from build123d import *

# Parameters (mm, degrees)
SKETCH1_W               = 95.2
SKETCH1_H               = 135.7
BOSS_EXTRUDE1_DEPTH     = 240
SKETCH3_W               = 228.6
SKETCH3_H               = 83.8
CUT_EXTRUDE1_DEPTH      = 124.3
FILLET1_R               = 1
SKETCH6_R               = 23.5
CUT_EXTRUDE2_DEPTH      = 140
SKETCH7_W               = 55
SKETCH7_H               = 45.7
BOSS_EXTRUDE2_DEPTH     = 8.3
SKETCH8_R               = 23.5
CUT_EXTRUDE3_DEPTH      = 295.494040687
SKETCH9_W               = 55
SKETCH9_H               = 45.7
BOSS_EXTRUDE3_DEPTH     = 8.3
SKETCH10_R              = 23.5
CUT_EXTRUDE4_DEPTH      = 298.512571163
CUT_EXTRUDE5_DEPTH      = 295.494040687
CUT_EXTRUDE5_DEPTH_BACK = 295.494040687
SKETCH11_R              = 4
SKETCH12_W              = 46
SKETCH12_H              = 10
BOSS_EXTRUDE4_DEPTH     = 2
SKETCH13_W              = 46
SKETCH13_H              = 10
BOSS_EXTRUDE5_DEPTH     = 2


with BuildPart() as part:
    # Sketch1 → Boss-Extrude1 (new body)
    with BuildSketch(Plane(origin=(0, 0, 0), x_dir=(0, 0, -1), z_dir=(1, 0, 0))):
        with Locations((47.6, 67.85)):
            Rectangle(SKETCH1_W, SKETCH1_H)
    extrude(amount=-BOSS_EXTRUDE1_DEPTH)

    # Sketch3 → Cut-Extrude1 (cut)
    with BuildSketch(Plane(origin=(0, 135.7, 0), x_dir=(1, 0, 0), z_dir=(0, 1, 0))):
        with Locations((-120, 47.6)):
            Rectangle(SKETCH3_W, SKETCH3_H)
    extrude(amount=-CUT_EXTRUDE1_DEPTH, mode=Mode.SUBTRACT)

    # Fillet1
    fillet1_edges = [part.edges().sort_by_distance(p)[0] for p in [
        (-240, 67.85, -95.2),
        (-240, 67.85, 0),
        (0, 67.85, -95.2),
        (0, 0, -47.6),
        (0, 67.85, 0),
        (-120, 0, -95.2),
        (-120, 0, 0),
        (-240, 0, -47.6),
    ]]
    fillet(fillet1_edges, radius=FILLET1_R)

    # Sketch6 → Cut-Extrude2 (cut)
    with BuildSketch(Plane.XY):
        with Locations((-120, 117.5)):
            Circle(SKETCH6_R)
    extrude(amount=-CUT_EXTRUDE2_DEPTH, mode=Mode.SUBTRACT)

    # Sketch7 → Boss-Extrude2 (add)
    with BuildSketch(Plane.XY):
        with Locations((-120, 112.85)):
            Rectangle(SKETCH7_W, SKETCH7_H)
    extrude(amount=BOSS_EXTRUDE2_DEPTH)

    # Sketch8 → Cut-Extrude3 (cut, through all)
    with BuildSketch(Plane(origin=(0, 0, -95.2), x_dir=(-1, 0, 0), z_dir=(0, 0, -1))):
        with Locations((120, 117.5)):
            Circle(SKETCH8_R)
    extrude(amount=-CUT_EXTRUDE3_DEPTH, mode=Mode.SUBTRACT)

    # Sketch9 → Boss-Extrude3 (add)
    with BuildSketch(Plane(origin=(0, 0, -95.2), x_dir=(-1, 0, 0), z_dir=(0, 0, -1))):
        with Locations((120, 112.85)):
            Rectangle(SKETCH9_W, SKETCH9_H)
    extrude(amount=BOSS_EXTRUDE3_DEPTH)

    # Sketch10 → Cut-Extrude4 (cut, through all)
    with BuildSketch(Plane.XY.offset(8.3)):
        with Locations((-120, 117.5)):
            Circle(SKETCH10_R)
    extrude(amount=-CUT_EXTRUDE4_DEPTH, mode=Mode.SUBTRACT)

    # Sketch11 → Cut-Extrude5 (cut, two sides: drawn at the far end of the back side and taken through both)
    with BuildSketch(Plane.XY.offset(-CUT_EXTRUDE5_DEPTH_BACK)):
        with Locations((-30, 128.7)):
            Circle(SKETCH11_R)
        with Locations((-210, 128.7)):
            Circle(SKETCH11_R)
    extrude(amount=CUT_EXTRUDE5_DEPTH + CUT_EXTRUDE5_DEPTH_BACK, mode=Mode.SUBTRACT)

    # Sketch12 → Boss-Extrude4 (add)
    with BuildSketch(Plane.XY.offset(8.3)):
        with Locations((-120, 97)):
            Rectangle(SKETCH12_W, SKETCH12_H)
    extrude(amount=BOSS_EXTRUDE4_DEPTH)

    # Sketch13 → Boss-Extrude5 (add)
    with BuildSketch(Plane(origin=(0, 0, -103.5), x_dir=(-1, 0, 0), z_dir=(0, 0, -1))):
        with Locations((120, 97)):
            Rectangle(SKETCH13_W, SKETCH13_H)
    extrude(amount=BOSS_EXTRUDE5_DEPTH)


solid = part.part
Geometry check sheet. Reference: the model listing, model coordinates, mm. A direction names the side the tool comes from. Coordinates: 2 decimals unless noted, no trailing zeros. Order: outer loops, then holes, each group sorted by start corner. A loop starts at its lowest first (then second) coordinate and runs counter-clockwise, first axis right, second up. Notation, with made-up numbers: M -12.5,38 L 28.5,38 A18 ccw 28.5,43 Z; hole C 68,-31.5 d9. An arc over 180 degrees is marked long. Use CSV: the item, a comma, the result in double quotes.
Item 1: Gauge pin test, flat ends, axial feed: pin 1 Ø9 at (y, z) = (123.5, -101) entering from +X; pin 2 Ø1 at (x, z) = (-111.5, -104) entering from +Y; pin 3 Ø6 at (x, y) = (-208.5, 94) entering from -Z. Record the tip position at first contact, or that the pin passes through.
Returned:
pin 1,"stops at x = -92.5"
pin 2,"stops at y = 102"
pin 3,"stops at z = -95.2"
Item 2: Cross-section at D-D on x = -217. Record the cut outline in (y, z).
Returned:
outline,"M 0,-94.2 A1 ccw 1,-95.2 L 135.7,-95.2 L 135.7,-89.5 L 11.4,-89.5 L 11.4,-5.7 L 135.7,-5.7 L 135.7,0 L 1,0 A1 ccw 0,-1 Z"
Item 3: Cross-section at A-A on y = 117.5. Record the cut outline in (x, z).
Returned:
outline,"M -240,-94.2 A1 ccw -239,-95.2 L -147.5,-95.2 L -147.5,-103.5 L -143.5,-103.5 L -143.5,-89.5 L -234.3,-89.5 L -234.3,-5.7 L -143.5,-5.7 L -143.5,8.3 L -147.5,8.3 L -147.5,0 L -239,0 A1 ccw -240,-1 Z; M -96.5,-103.5 L -92.5,-103.5 L -92.5,-95.2 L -1,-95.2 A1 ccw 0,-94.2 L 0,-1 A1 ccw -1,0 L -92.5,0 L -92.5,8.3 L -96.5,8.3 L -96.5,-5.7 L -5.7,-5.7 L -5.7,-89.5 L -96.5,-89.5 Z"
Item 4: Cross-section at B-B on x = -30. Record the cut outline in (y, z), then the cut area to 3 significant figures.
Returned:
outline,"M 0,-94.2 A1 ccw 1,-95.2 L 124.7,-95.2 L 124.7,-89.5 L 11.4,-89.5 L 11.4,-5.7 L 124.7,-5.7 L 124.7,0 L 1,0 A1 ccw 0,-1 Z; M 132.7,-95.2 L 135.7,-95.2 L 135.7,-89.5 L 132.7,-89.5 Z; M 132.7,-5.7 L 135.7,-5.7 L 135.7,0 L 132.7,0 Z"
area,"2,410 mm2"
Item 5: Tool access check on faces 4 (the flat face through (-5.7, 74, -47)), 5 (the flat face through (-147.5, 113, 4)), 6 (the cylindrical face through (-120.808, 94.014, -96.402)). Record the directions out of +Z, -Z, +X, -X, +Y, -Y that give a thin tool (end or side, any length) a straight path to the whole face; none if there is none.
Returned:
face 4,"+Y"
face 5,"+Z, -X, +Y, -Y"
face 6,"none"
Item 6: Thickness scan on line 1 along Z through (x, y) = (-38, 53.5); line 2 along X through (y, z) = (65, -27.5); line 3 along Y through (x, z) = (-30, -4.3). Record the ranges inside material, lowest first.
Returned:
line 1,"z = -95.2 to -89.5, -5.7 to 0"
line 2,"x = -240 to -234.3, -5.7 to 0"
line 3,"y = 0 to 124.7, 132.7 to 135.7"
Item 7: Cross-section at C-C on y = 31.5. Record the cut outline in (x, z), then the cut area to 3 significant figures.
Returned:
outline,"M -240,-94.2 A1 ccw -239,-95.2 L -1,-95.2 A1 ccw 0,-94.2 L 0,-1 A1 ccw -1,0 L -239,0 A1 ccw -240,-1 Z; hole M -234.3,-89.5 L -5.7,-89.5 L -5.7,-5.7 L -234.3,-5.7 Z"
area,"3,690 mm2"
Item 8: Mould release check, pull along Y, two halves, no side actions. Record for faces 1 (the cylindrical face through (-30.867, 124.795, -92.39)), 2 (the flat face through (-122, 11.4, -48)), 3 (the flat face through (-240, 69, -47)): pulls with the +Y half, pulls with the -Y half, needs draft (parallel to the pull), parting line crosses it, or undercut.
Returned:
face 1,"undercut"
face 2,"pulls with the +Y half"
face 3,"needs draft"
